Here's the drawing with two shaded views (mm, measured from the low corner). I have some questions. Coordinates: 2 decimals unless noted, no trailing zeros. Write each loop counter-clockwise with the first axis right and the second up, starting at its lowest first coordinate (ties: lowest second). Pieces come first, ordered by that corner, then holes.
Item 1: If we section it at C-C (y = 0.2): Please give me the cut outline in (x, z), then the cut area to 3 significant figures.
Item 2: If we section it at B-B (z = 18.25): Please give me the cut outline in (x, y), then the cut area to 3 significant figures.
Item 3: If I drill on line 1 (Z direction, x = 25, y = 0.35); line 2 (X direction, y = 0.55, z = 18.25); line 3 (X direction, y = 0.3, z = 19.5), over which ranges is the centre line in solid material (lowest first)?
Item 4: If we section it at A-A (x = 25): Please give me the cut outline in (y, z).
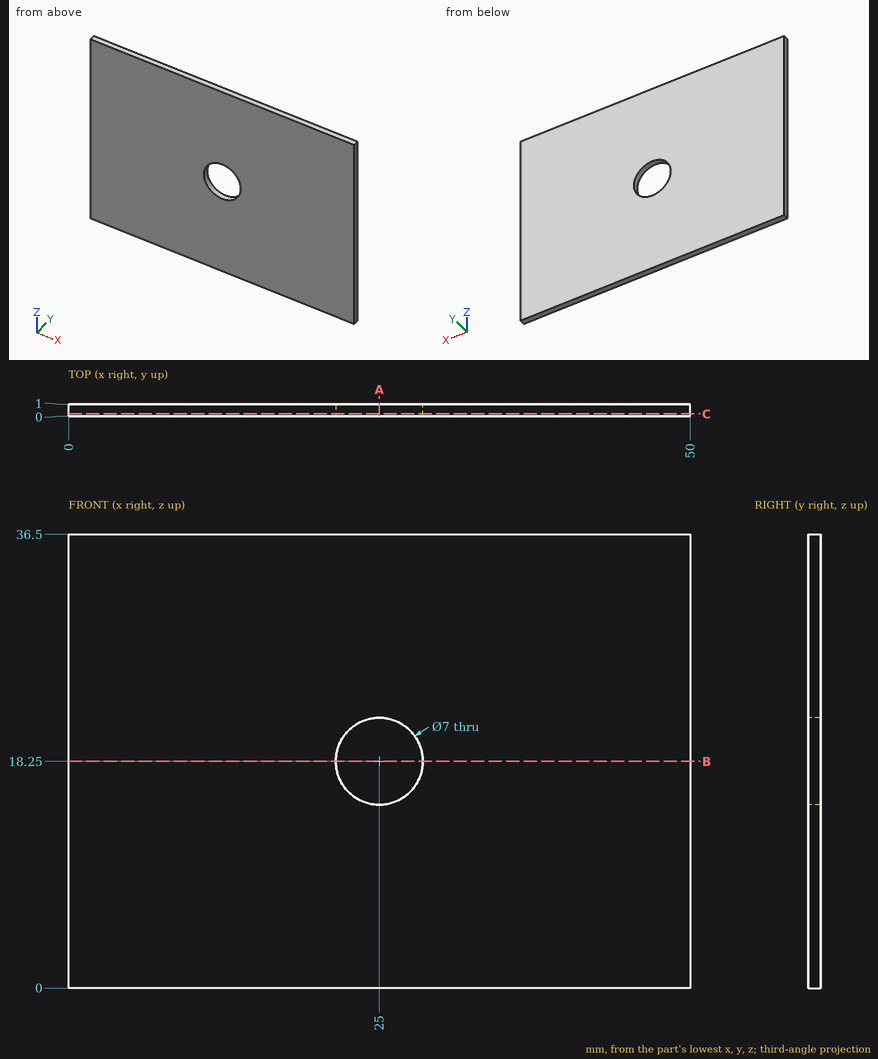
Answer list:
1. outline: (0, 0) - (50, 0) - (50, 36.5) - (0, 36.5) - close; hole circle Ø7 at (25, 18.25)
1. area: 1,790 mm2
2. outline: (0, 0) - (21.5, 0) - (21.5, 1) - (0, 1) - close; (28.5, 0) - (50, 0) - (50, 1) - (28.5, 1) - close
2. area: 43.0 mm2
3. line 1: z = 0 to 14.75, 21.75 to 36.5
3. line 2: x = 0 to 21.5, 28.5 to 50
3. line 3: x = 0 to 21.73, 28.27 to 50
4. outline: (0, 0) - (1, 0) - (1, 14.75) - (0, 14.75) - close; (0, 21.75) - (1, 21.75) - (1, 36.5) - (0, 36.5) - close
